The model under review builds one solid part; all positions refer to its coordinate system, in mm. A direction names the side the tool comes from. Give positions to 0.01 mm unless a question says otherwise; leave off trailing zeros. Order: outer loops, then holes, each group sorted by start corner. A loop starts at its lowest first (then second) coordinate and runs counter-clockwise, first axis right, second up. Notation, with made-up numbers: (35.5, 8) - (57.5, 8) arc R28 cw to (57.5, 40) - close; hole circle Ø5 at (48, -35). An arc over 180 degrees is marked (long way). Write item = value, one per line. Start each with the question number.
1. Wall thickness on probe 1 along Y at (x, z) = (-0.75, -1.75); probe 2 along Z at (x, y) = (0.25, -2.5); probe 3 along X at (y, z) = (-6.5, 0.15): over which ranges is each line inside the solid? List them lowest first.
2. For P1, Ø6, axis at x = 1, y = 0.5, coming from the -Z side; P2, Ø2, axis at x = -1.5, z = -0.5, coming from the -Y side; P3, Ø1.3, axis at x = 2, z = 0.5, coming from the +Y side, all flat-tipped, find the tip position at first contact; note any pin that passes through.
3. We need section A-A, the plane z = 0. Give the boundary of the cut face in (x, y).
4. We need section B-B, the plane y = 6.5. Give the boundary of the cut face in (x, z).
5. We need section C-C, the plane x = 3.75. Give the boundary of the cut face in (y, z), and give its area (3 significant figures).
6. We need section D-D, the plane y = -1.75. Give the boundary of the cut face in (x, z), and give its area (3 significant figures).
7. Machinability: for faces 1 (the flat face through (0, 0, 2.25)), 2 (the flat face through (0, 0, -2.25)), 3 (the flat face through (-6, 0, 0)), 4 (the flat face through (0, -6, 0)), 5 (the flat face through (0, 6, 0)), which of the approach directions +Z, -Z, +X, -X, +Y, -Y give a long, thin tool a straight path to every point of the face, cutting with its end or side? Answer none if there is none.
from build123d import *

# Parameters (mm, degrees)
SKETCH1_W           = 12
SKETCH1_H           = 12
BOSS_EXTRUDE1_DEPTH = 2.25
SKETCH1_3_W         = 7
SKETCH1_3_H         = 15
BOSS_EXTRUDE2_DEPTH = 3
FILLET1_R           = 0.5


with BuildPart() as part:
    # Sketch1 → Boss-Extrude1 (new, symmetric)
    with BuildSketch(Plane.XY):
        Rectangle(SKETCH1_W, SKETCH1_H)
    extrude(amount=BOSS_EXTRUDE1_DEPTH, both=True)

    # Sketch1<3> → Boss-Extrude2 (add, symmetric)
    with BuildSketch(Plane.XY):
        with Locations((9.5, 0)):
            Rectangle(SKETCH1_3_W, SKETCH1_3_H)
    extrude(amount=BOSS_EXTRUDE2_DEPTH, both=True)

    # Fillet1
    fillet1_edges = [part.edges().sort_by_distance(p)[0] for p in [
        (13, 0, -3),
        (13, -7.5, 0),
        (9.5, 7.5, -3),
        (13, 7.5, 0),
        (6, 0, 3),
        (6, 7.5, 0),
        (9.5, -7.5, 3),
        (6, -7.5, 0),
        (13, 0, 3),
        (9.5, 7.5, 3),
        (9.5, -7.5, -3),
        (6, 0, -3),
    ]]
    fillet(fillet1_edges, radius=FILLET1_R)


solid = part.part
Model answer:
q1.probe_1 = -6 to 6
q1.probe_2 = -2.25 to 2.25
q1.probe_3 = 6 to 13
q2.P1 = -2.25
q2.P2 = -6
q2.P3 = 6
q3.outline = (-6, -6) - (6, -6) - (6, -7) arc R0.5 ccw to (6.5, -7.5) - (12.5, -7.5) arc R0.5 ccw to (13, -7) - (13, 7) arc R0.5 ccw to (12.5, 7.5) - (6.5, 7.5) arc R0.5 ccw to (6, 7) - (6, 6) - (-6, 6) - close
q4.outline = (6, -2.5) arc R0.5 ccw to (6.5, -3) - (12.5, -3) arc R0.5 ccw to (13, -2.5) - (13, 2.5) arc R0.5 ccw to (12.5, 3) - (6.5, 3) arc R0.5 ccw to (6, 2.5) - close
q5.outline = (-6, -2.25) - (6, -2.25) - (6, 2.25) - (-6, 2.25) - close
q5.area = 54.0 mm2
q6.outline = (-6, -2.25) - (6, -2.25) - (6, -2.5) arc R0.5 ccw to (6.5, -3) - (12.5, -3) arc R0.5 ccw to (13, -2.5) - (13, 2.5) arc R0.5 ccw to (12.5, 3) - (6.5, 3) arc R0.5 ccw to (6, 2.5) - (6, 2.25) - (-6, 2.25) - close
q6.area = 95.8 mm2
q7.face_1 = +Z, -X, +Y, -Y
q7.face_2 = -Z, -X, +Y, -Y
q7.face_3 = +Z, -Z, -X, +Y, -Y
q7.face_4 = +Z, -Z, -X, -Y
q7.face_5 = +Z, -Z, -X, +Y
